The listing builds one solid part. Answer for the finished solid, in the listing's coordinates (mm). Face numbers are marked on the shaded views. A direction names the side the tool comes from. Give positions to 0.01 mm unless a question says otherwise; leave off trailing zeros. Write each loop counter-clockwise with the first axis right and the second up, starting at its lowest first coordinate (ties: lowest second). Pieces come first, ordered by that corner, then holes. Notation, with made-up numbers: (71.5, 24.5) -> (130.5, 24.5) arc R21 ccw to (130.5, 62.5) -> close; hole circle Ø5 at (-26.75, -3.5). An arc over 180 degrees is marked (long way). One line per question, with ' | ' between items.
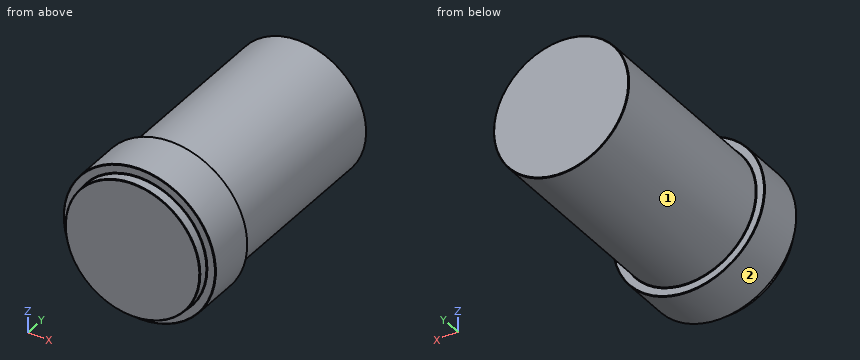
from build123d import *

# Parameters (mm, degrees)
SKETCH1_R           = 22.5
BOSS_EXTRUDE1_DEPTH = 65
SKETCH2_R           = 25.3
BOSS_EXTRUDE2_DEPTH = 16.4
SKETCH3_R           = 22.4
BOSS_EXTRUDE3_DEPTH = 3.5
CHAMFER1_SIZE       = 0.2


with BuildPart() as part:
    # Sketch1 → Boss-Extrude1 (new body)
    with BuildSketch(Plane(origin=(0, 0, 0), x_dir=(1, 0, 0), z_dir=(0, 1, 0))):
        with Locations(Location((0, 0, 0), (0, 0, 270))):
            Circle(SKETCH1_R)
    extrude(amount=BOSS_EXTRUDE1_DEPTH)

    # Sketch2 → Boss-Extrude2 (add)
    with BuildSketch(Plane.XZ):
        with Locations(Location((0, 0, 0), (0, 0, 270))):
            Circle(SKETCH2_R)
    extrude(amount=BOSS_EXTRUDE2_DEPTH)

    # Sketch3 → Boss-Extrude3 (add)
    with BuildSketch(Plane.XZ.offset(16.4)):
        with Locations(Location((0, 0, 0), (0, 0, 270))):
            Circle(SKETCH3_R)
    extrude(amount=BOSS_EXTRUDE3_DEPTH)

    # Chamfer1
    chamfer1_edges = [part.edges().sort_by_distance(p)[0] for p in [
        (0, -19.9, 22.4),
        (0, 65, -22.5),
        (0, 0, -22.5),
        (0, 0, 25.3),
        (0, -16.4, 25.3),
        (0, -16.4, 22.4),
    ]]
    chamfer(chamfer1_edges, length=CHAMFER1_SIZE)


solid = part.part
Item 1: Find section A-A (x = 0). Write down the section's boundary in (y, z), then the cut area to 3 significant figures.
Answers below:
outline: (-19.9, -22.2) -> (-19.7, -22.4) -> (-16.6, -22.4) -> (-16.4, -22.6) -> (-16.4, -25.1) -> (-16.2, -25.3) -> (-0.2, -25.3) -> (0, -25.1) -> (0, -22.7) -> (0.2, -22.5) -> (64.8, -22.5) -> (65, -22.3) -> (65, 22.3) -> (64.8, 22.5) -> (0.2, 22.5) -> (0, 22.7) -> (0, 25.1) -> (-0.2, 25.3) -> (-16.2, 25.3) -> (-16.4, 25.1) -> (-16.4, 22.6) -> (-16.6, 22.4) -> (-19.7, 22.4) -> (-19.9, 22.2) -> close | area: 3,910 mm²
Item 2: A tool of negligible diameter and unlimited length cuts with its end or side. For the marked faces 1 and 2, from which of +Z, -Z, +X, -X, +Y, -Y can it reach the whole face along a straight path? Write none if from no direction.
Answers below:
face 1: +Y | face 2: +Y, -Y
Item 3: Consider line 1 (Z direction, x = -3, y = 22); line 2 (Z direction, x = 3.5, y = 9.5); line 3 (X direction, y = -8, z = 11). Determine where each line is inside the solid, lowest interval first. Write a range as [from, to].
Answers below:
line 1: [-22.3, 22.3] | line 2: [-22.23, 22.23] | line 3: [-22.78, 22.78]
Item 4: Find section B-B (z = 0). Write down the section's boundary in (x, y), then the cut area to 3 significant figures.
Answers below:
outline: (-25.3, -16.2) -> (-25.1, -16.4) -> (-22.6, -16.4) -> (-22.4, -16.6) -> (-22.4, -19.7) -> (-22.2, -19.9) -> (22.2, -19.9) -> (22.4, -19.7) -> (22.4, -16.6) -> (22.6, -16.4) -> (25.1, -16.4) -> (25.3, -16.2) -> (25.3, -0.2) -> (25.1, 0) -> (22.7, 0) -> (22.5, 0.2) -> (22.5, 64.8) -> (22.3, 65) -> (-22.3, 65) -> (-22.5, 64.8) -> (-22.5, 0.2) -> (-22.7, 0) -> (-25.1, 0) -> (-25.3, -0.2) -> close | area: 3,910 mm²
Item 5: Flat-ended cylindrical pins translate along their axes: pin 1 (6 mm diameter, centred on y = 26.5, z = 8, fed in from -X); pin 2 (3 mm diameter, centred on x = 19.5, y = -7.5, fed in from -Z); pin 3 (1 mm diameter, centred on x = -14, y = 32.5, fed in from -Z). Find the tip coordinate at first contact, or state that the pin passes through.
Answers below:
pin 1: x = -21.94 | pin 2: z = -17.78 | pin 3: z = -18
